Could you check a few things on this model? Use its own coordinates, in mm. A direction names the side the tool comes from. Round coordinates to 2 decimals unless told otherwise and drop trailing zeros. Loops run counter-clockwise (first coordinate to the right, second up) from the corner with the lowest first, then second, coordinate; pieces in that order, holes last. Notation, with made-up numbers: (24, -24.75) - (65, -24.75) arc R35 ccw to (65, 14.25) - close; hole circle Ø7 at (37.25, -10.75). An arc over 180 degrees is marked (long way). Put each result on its own line as item: value. Start each with the question number.
from build123d import *

# Parameters (mm, degrees)
PAD015_DEPTH            = 0.8
SKETCH029_W             = 7
SKETCH029_H             = 7
PAD017_DEPTH            = 1.5
SKETCH028_R             = 1.5
HOLE008_DEPTH           = 25
SKETCH022_R             = 10.5
PAD020_DEPTH            = 3.5
PAD021_DEPTH            = 4.5
PAD021_TAPER            = 15
SKETCH023_R             = 2
HOLE010_DEPTH           = 25
SKETCH036_R             = 10.5
POCKET003_DEPTH         = 5
BODY009_PLACEMENT_ANGLE = 180


with BuildPart() as as5600:
    # Sketch027 → Pad015 (new body, symmetric)
    with BuildSketch(Plane.XY):
        with BuildLine():
            Line((-11.5, 8.5), (-11.5, -8.5))
            ThreePointArc((-11.5, -8.5), (-10.62132, -10.62132), (-8.5, -11.5))
            Line((-8.5, -11.5), (8.5, -11.5))
            ThreePointArc((8.5, -11.5), (10.62132, -10.62132), (11.5, -8.5))
            Line((11.5, -8.5), (11.5, 8.5))
            ThreePointArc((11.5, 8.5), (10.62132, 10.62132), (8.5, 11.5))
            Line((8.5, 11.5), (-8.5, 11.5))
            ThreePointArc((-8.5, 11.5), (-10.62132, 10.62132), (-11.5, 8.5))
        make_face()
    extrude(amount=PAD015_DEPTH, both=True)

    # Sketch029 → Pad017 (join)
    with BuildSketch(Plane.XY.offset(0.8)):
        with BuildLine():
            ThreePointArc((-5, 8.5), (-6.5, 7), (-5, 5.5))
            Line((-5, 5.5), (5, 5.5))
            ThreePointArc((5, 5.5), (6.5, 7), (5, 8.5))
            Line((-5, 8.5), (5, 8.5))
        make_face()
        with BuildLine():
            ThreePointArc((-3.5, -4.5), (-5, -6), (-3.5, -7.5))
            Line((-3.5, -7.5), (3.5, -7.5))
            ThreePointArc((3.5, -7.5), (5, -6), (3.5, -4.5))
            Line((-3.5, -4.5), (3.5, -4.5))
        make_face()
        Rectangle(SKETCH029_W, SKETCH029_H)
        with BuildLine():
            ThreePointArc((-8, -5.5), (-6.8, -6.7), (-5.6, -5.5))
            Line((-5.6, -5.5), (-5.6, 4))
            ThreePointArc((-5.6, 4), (-6.8, 5.2), (-8, 4))
            Line((-8, -5.5), (-8, 4))
        make_face()
        with BuildLine():
            ThreePointArc((6.8, 3.38), (5.8, 4.38), (4.8, 3.38))
            Line((4.8, 3.38), (4.8, -3.38))
            ThreePointArc((4.8, -3.38), (5.8, -4.38), (6.8, -3.38))
            Line((6.8, 3.38), (6.8, -3.38))
        make_face()
    extrude(amount=PAD017_DEPTH)

    # Sketch028 (on Face10 of Pad015) → Hole008 (cut)
    with BuildSketch(Plane.XY.offset(0.8)):
        with Locations((-8.5, 8.5)):
            Circle(SKETCH028_R)
        with Locations((8.5, 8.5)):
            Circle(SKETCH028_R)
        with Locations((-8.5, -8.5)):
            Circle(SKETCH028_R)
        with Locations((8.5, -8.5)):
            Circle(SKETCH028_R)
    extrude(amount=-HOLE008_DEPTH, mode=Mode.SUBTRACT)


with BuildPart() as as5600_1:
    # Body001 placement: moved
    add(as5600.part.moved(Location((0, 0, -7.7))))


with BuildPart() as obj1:
    # Sketch022 → Pad020 (new body)
    with BuildSketch(Plane.XY):
        with BuildLine():
            ThreePointArc((13.586881, 20.251823), (0, 30.3), (-13.586881, 20.251823))
            ThreePointArc((-17.728491, 11.256137), (-15.355357, 15.614788), (-13.586881, 20.251823))
            ThreePointArc((-17.728491, 11.256137), (-20.699674, -3.538854), (-12.982142, -16.506483))
            ThreePointArc((-6.502297, -26.893782), (-8.833051, -21.132971), (-12.982142, -16.506483))
            ThreePointArc((-6.502297, -26.893782), (0, -32.15), (6.502297, -26.893782))
            ThreePointArc((12.982142, -16.506483), (8.833051, -21.132971), (6.502297, -26.893782))
            ThreePointArc((12.982142, -16.506483), (20.699674, -3.538854), (17.728491, 11.256137))
            ThreePointArc((13.586881, 20.251823), (15.355357, 15.614788), (17.728491, 11.256137))
        make_face()
        Circle(SKETCH022_R, mode=Mode.SUBTRACT)
    extrude(amount=PAD020_DEPTH)

    # Sketch026 (on Face11 of Pad020) → Pad021 (join)
    with BuildSketch(Plane.XY.offset(3.5)):
        with BuildLine():
            Line((-14.8, 11), (-14.8, -11))
            ThreePointArc((-14.8, -11), (-13.628427, -13.828427), (-10.8, -15))
            Line((-10.8, -15), (10.8, -15))
            ThreePointArc((10.8, -15), (13.628427, -13.828427), (14.8, -11))
            Line((14.8, -11), (14.8, 11))
            ThreePointArc((14.8, 11), (13.628427, 13.828427), (10.8, 15))
            Line((10.8, 15), (-10.8, 15))
            ThreePointArc((-10.8, 15), (-13.628427, 13.828427), (-14.8, 11))
        make_face()
    extrude(amount=PAD021_DEPTH, taper=PAD021_TAPER)

    # Sketch023 → Hole010 (cut)
    with BuildSketch(Plane.XY):
        with Locations((0, -25.5)):
            Circle(SKETCH023_R)
        with Locations((-8, 21.5)):
            Circle(SKETCH023_R)
        with Locations((8, 21.5)):
            Circle(SKETCH023_R)
        with Locations((0, -25.5)):
            Circle(SKETCH023_R)
        with Locations((-8, 21.5)):
            Circle(SKETCH023_R)
        with Locations((8, 21.5)):
            Circle(SKETCH023_R)
    extrude(amount=HOLE010_DEPTH, mode=Mode.SUBTRACT)

    # Sketch036 → Pocket003 (cut)
    with BuildSketch(Plane.XY):
        Circle(SKETCH036_R)
    extrude(amount=POCKET003_DEPTH, mode=Mode.SUBTRACT)


with BuildPart() as obj1_1:
    # Body009 placement: moved
    add(obj1.part.moved(Location((0, 0, -0.5))).rotate(Axis((0, 0, -0.5), (0, 1, 0)), BODY009_PLACEMENT_ANGLE))

    # Cut009: cut AS5600
    add(as5600_1.part, mode=Mode.SUBTRACT)


solid = obj1_1.part
Item 1: Suppose I cut it at C-C, the plane x = -17. List the corners of the cut face in (y, z) for me, then the cut area to 3 significant figures.
Item 2: Suppose I cut it at D-D, the plane y = 16. List the corners of the cut face in (x, z) for me.
Item 3: On a 3-axis mill with a long thin cutter (end or side, diameter ignored), from which of +Z, -Z, +X, -X, +Y, -Y can I reach the whole of each face in a straight line? I mean faces 1 (the face through (-5, 0, -5.5)), 2 (the face through (-8, -1, -6)), 3 (the face through (10.64, 10.6, -7.69)). Say none if no direction works.
Item 4: I need wall thicknesses on line 1 (X direction, y = 6.5, z = -7.75); line 2 (X direction, y = 21.5, z = -1.5); line 3 (Y direction, x = -6, z = -6.5). Which ranges of each line are inside material? Lowest first, please. Write a range as from..to.
Item 5: Suppose I cut it at A-A, the plane x = 0. Count the separate pieces of the cut face and the enclosed holes in it, then the cut area to 3 significant figures.
Item 6: Suppose I cut it at B-B, the plane z = -3.25. List the corners of the cut face in (x, y) for me.
Item 7: Thinking about a two-plate mould opening in Y: for faces 4 (the face through (13.22, -13.37, -6.28)), 5 (the face through (-11.5, 0, -8)), 6 (the face through (-15.326, 15.678, -2.226)), which applies, released by +Y, released by -Y, zero draft, split by the parting line, or undercut?
Item 8: Will these pins go through, and if not, where does the flat tip stop? P1, Ø1.1, axis at x = -0.5, z = -6.5, coming from the +Y side; P2, Ø1.8, axis at x = -3.5, z = -7.5, coming from the -Y side; P3, Ø0.7, axis at x = 0.5, z = -6, coming from the -Y side; P4, Ø1.5, axis at x = -14, y = 22, coming from the +Z side.
Numbers:
1. outline: (-12.33, -4) - (12.45, -4) - (12.45, -0.5) - (-12.33, -0.5) - close
1. area: 86.7 mm^2
2. outline: (-15.18, -4) - (15.18, -4) - (15.18, -0.5) - (-15.18, -0.5) - close
3. face 1: +Z
3. face 2: +Z, -Z
3. face 3: -Z
4. line 1: -13.8..-11.5, 11.5..13.8
4. line 2: -13.14..-10, -6..6, 10..13.14
4. line 3: -14.33..-6.39, 4.89..5.88, 8.12..14.33
5. separate pieces: 5
5. enclosed holes: 0
5. area: 174 mm^2
6. outline: (-17.73, 11.26) arc R21 ccw to (-12.98, -16.51) arc R18.02 cw to (-6.5, -26.89) arc R6.65 ccw to (6.5, -26.89) arc R18.02 cw to (12.98, -16.51) arc R21 ccw to (17.73, 11.26) arc R37 cw to (13.59, 20.25) arc R14.21 ccw to (-13.59, 20.25) arc R37 cw to start; hole circle Ø21 at (0, 0); hole circle Ø4 at (-8, 21.5); hole circle Ø4 at (0, -25.5); hole circle Ø4 at (8, 21.5)
7. face 4: released by -Y
7. face 5: undercut
7. face 6: released by +Y
8. P1: y = 14.48
8. P2: y = -14.3
8. P3: y = -14.56
8. P4: through
